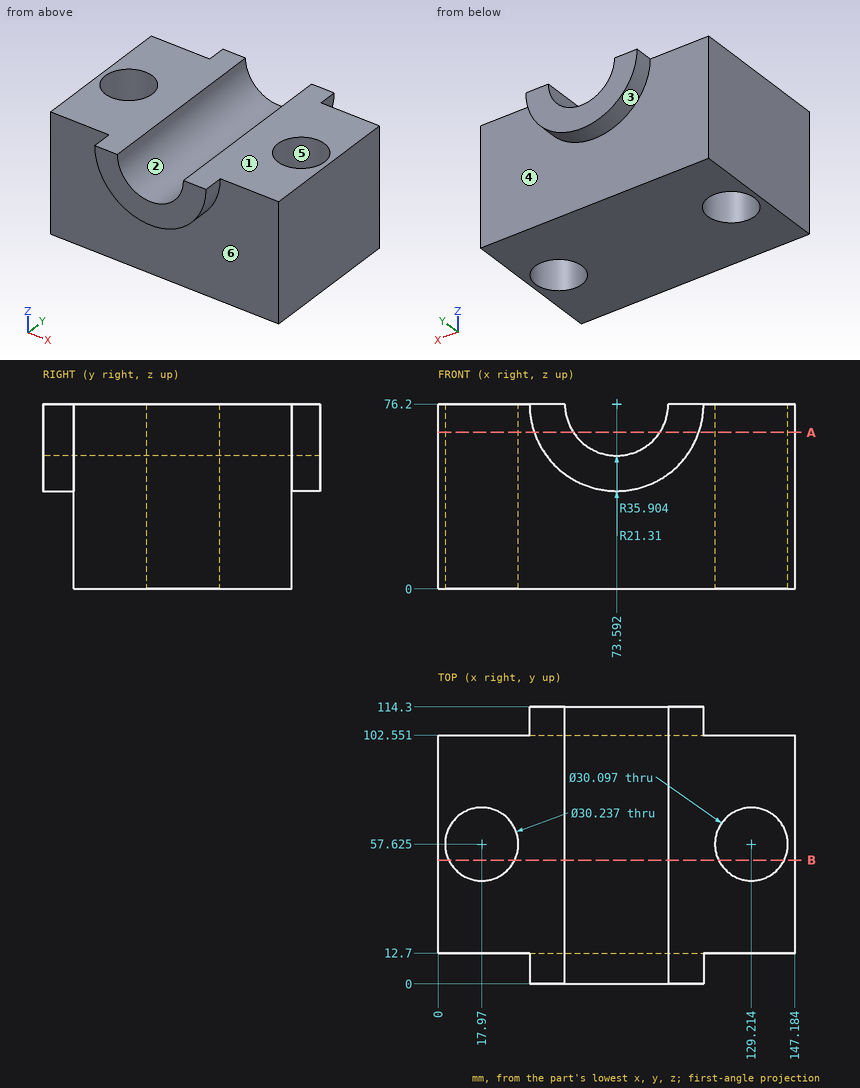
Verification items for this drawing (mm, ordinates from the low corner). A direction names the side the tool comes from. Coordinates: 2 decimals unless noted, no trailing zeros. Loops run counter-clockwise (first coordinate to the right, second up) from the corner with the lowest first, then second, coordinate; pieces in that order, holes last. Notation, with made-up numbers: (-23.5, -20.5) - (35.5, -20.5) arc R25 ccw to (35.5, -5.5) - close; hole circle Ø8 at (-1, 40). An arc over 180 degrees is marked (long way). Answer as a JSON object with one key per item and string values.
(1) Cross-section at B-B, the plane y = 51. Record the boundary of the cut face in (x, z) (1 decimal), then the cut area to 3 significant figures.
Response:
{"outline": "(0, 0) - (4.4, 0) - (4.4, 76.2) - (0, 76.2) - close; (31.6, 0) - (115.7, 0) - (115.7, 76.2) - (94.9, 76.2) arc R21.3 cw to (52.3, 76.2) - (31.6, 76.2) - close; (142.7, 0) - (147.2, 0) - (147.2, 76.2) - (142.7, 76.2) - close", "area": "6,370 mm²"}
(2) Go/stop test with flat-tipped pins: pin 1 Ø8 at (y, z) = (91.5, 33) entering from -X; pin 2 Ø1 at (x, z) = (22, 26.5) entering from +Y; pin 3 Ø6 at (x, y) = (71, 71.5) entering from +Z. Record where each tip stops, or that it passes through.
Response:
{"pin 1": "stops at x = 0", "pin 2": "stops at y = 102.55", "pin 3": "stops at z = 55.64"}
(3) Access from +Z, -Z, +X, -X, +Y, -Y to the whole of each face (thin tool, end or side, straight path). Record for the marked faces 4, 5 and 6.
Response:
{"face 4": "-Z, +Y", "face 5": "+Z, -Z", "face 6": "-Z, -Y"}
(4) Cross-section at A-A, the plane z = 64.5. Count the separate pieces of the cut face and the enclosed holes in it, then the cut area to 3 significant figures.
Response:
{"separate pieces": "2", "enclosed holes": "2", "area": "9,380 mm²"}
(5) Mould release check, pull along X, two halves, no side actions. Record for the marked faces 1, 2 and 3: pulls with the +X half, pulls with the -X half, needs draft (parallel to the pull), parting line crosses it, or undercut.
Response:
{"face 1": "needs draft", "face 2": "undercut", "face 3": "parting line crosses it"}
(6) Scan lines: line 1 along X through (y, z) = (58, 43) (1 decimal); line 2 along X through (y, z) = (68, 6) (1 decimal); line 3 along Y through (x, z) = (81, 26.5). Record each from-to range of solid material in increasing order.
Response:
{"line 1": "x = 0 to 2.9, 33.1 to 114.2, 144.3 to 147.2", "line 2": "x = 0 to 7, 29 to 118.3, 140.1 to 147.2", "line 3": "y = 12.7 to 102.55"}
